```python
from build123d import *

# Parameters (mm, degrees)
SKETCH1_W           = 6.758532652
SKETCH1_H           = 42
SKETCH1_W_2         = 6
SKETCH1_W_3         = 6.758532653
BOSS_EXTRUDE1_DEPTH = 6


with BuildPart() as part:
    # Sketch1 → Boss-Extrude1 (new body)
    with BuildSketch(Plane(origin=(0, 0, 0), x_dir=(1, 0, 0), z_dir=(0, 1, 0))):
        Polygon((-88.584070796, 61.946902655), (-88.584070796, -148.053097345), (121.415929204, -148.053097345), (121.415929204, 61.946902655), (115.415929204, 61.946902655), (115.415929204, 67.946902655), (85.415929204, 67.946902655), (85.415929204, 61.946902655), (65.915929204, 61.946902655), (65.915929204, 67.946902655), (35.915929204, 67.946902655), (35.915929204, 61.946902655), (-3.084070796, 61.946902655), (-3.084070796, 67.946902655), (-33.084070796, 67.946902655), (-33.084070796, 61.946902655), (-52.584070796, 61.946902655), (-52.584070796, 67.946902655), (-82.584070796, 67.946902655), (-82.584070796, 61.946902655), align=None)
        with Locations((-79.20480447, -1.053097345)):
            Rectangle(SKETCH1_W, SKETCH1_H, mode=Mode.SUBTRACT)
        with Locations((-79.584070796, -85.053097345)):
            Rectangle(SKETCH1_W_2, SKETCH1_H, mode=Mode.SUBTRACT)
        with Locations((112.036662878, -1.053097345)):
            Rectangle(SKETCH1_W_3, SKETCH1_H, mode=Mode.SUBTRACT)
        with Locations((112.415929204, -85.053097345)):
            Rectangle(SKETCH1_W_2, SKETCH1_H, mode=Mode.SUBTRACT)
    extrude(amount=BOSS_EXTRUDE1_DEPTH)


solid = part.part
```
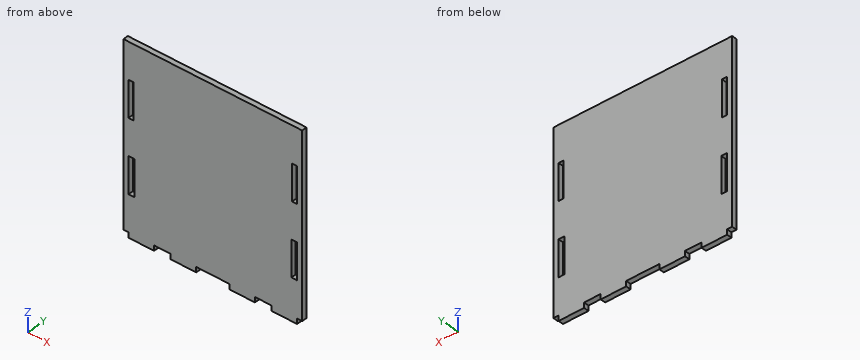
Build history of the part. All positions in model axes, mm. Give positions to 0.01 mm unless a question says otherwise; leave off trailing zeros. Loops run counter-clockwise (first coordinate to the right, second up) from the corner with the lowest first, then second, coordinate; pieces in that order, holes last.
Item 1: Drill centre lines: line 1 (X direction, y = 4.5, z = 98); line 2 (X direction, y = 4.75, z = 20.5); line 3 (Z direction, x = 112.5, y = 5.3). Where is each one in solid material? Low to high.
Answers follow:
line 1: x = -88.58 to -82.58, -76.58 to 109.42, 115.42 to 121.42
line 2: x = -88.58 to -82.58, -75.83 to 108.66, 115.42 to 121.42
line 3: z = -67.95 to -19.95, 22.05 to 64.05, 106.05 to 148.05
Item 2: Slice it at B-B, the plane y = 2.8. Give the number of separate pieces and of enclosed holes in the cut face, and give its area (3 significant figures).
Answers follow:
separate pieces: 1
enclosed holes: 4
area: 43,700 mm2
Item 3: Slice it at A-A, the plane z = 95. List the corners of the cut face in (x, y).
Answers follow:
outline: (-88.58, 0) - (-82.58, 0) - (-82.58, 6) - (-88.58, 6) - close; (-76.58, 0) - (109.42, 0) - (109.42, 6) - (-76.58, 6) - close; (115.42, 0) - (121.42, 0) - (121.42, 6) - (115.42, 6) - close
Item 4: Flat gauge pins, fed straight in: pin 1 (3 mm diameter, centred on y = 2.5, z = -63.5, fed in from +X); pin 2 (1.8 mm diameter, centred on y = 2.5, z = -66, fed in from -X); pin 3 (3 mm diameter, centred on x = -46, y = 3, fed in from -Z). Where does each tip first touch, or does it go through?
Answers follow:
pin 1: stops at x = 115.42
pin 2: stops at x = -82.58
pin 3: stops at z = -61.95
Item 5: Slice it at C-C, the plane z = -1. List the corners of the cut face in (x, y).
Answers follow:
outline: (-88.58, 0) - (-82.58, 0) - (-82.58, 6) - (-88.58, 6) - close; (-75.83, 0) - (108.66, 0) - (108.66, 6) - (-75.83, 6) - close; (115.42, 0) - (121.42, 0) - (121.42, 6) - (115.42, 6) - close
Item 6: Slice it at D-D, the plane x = 78.5. List the corners of the cut face in (y, z).
Answers follow:
outline: (0, -61.95) - (6, -61.95) - (6, 148.05) - (0, 148.05) - close
